```python
from build123d import *

# Parameters (mm, degrees)
SKETCH_1_W          = 56
SKETCH_1_H          = 56
EXTRUDE_1_DEPTH     = 55
SKETCH_2_W          = 9
SKETCH_2_H          = 9
CUT_EXTRUDE_1_DEPTH = 49
FILLET_1_R          = 2
SKETCH_3_R          = 19.1
EXTRUDE_2_DEPTH     = 1.6
SKETCH_4_R          = 3.175
EXTRUDE_3_DEPTH     = 18
SKETCH_5_R          = 2.5
CUT_EXTRUDE_2_DEPTH = 18
CHAMFER_1_SIZE      = 0.5


with BuildPart() as part:
    # Эскиз1 → Вытянуть1 (new body)
    with BuildSketch(Plane.XY):
        with Locations((28, 28)):
            Rectangle(SKETCH_1_W, SKETCH_1_H)
    extrude(amount=EXTRUDE_1_DEPTH)

    # Эскиз2 → Вырез-Вытянуть1 (cut)
    with BuildSketch(Plane(origin=(0, 0, 0), x_dir=(-1, 0, 0), z_dir=(0, 0, -1))):
        with Locations((-51.5, 51.5)):
            Rectangle(SKETCH_2_W, SKETCH_2_H)
        with Locations((-4.5, 51.5)):
            Rectangle(SKETCH_2_W, SKETCH_2_H)
        with Locations((-4.5, 4.5)):
            Rectangle(SKETCH_2_W, SKETCH_2_H)
        with Locations((-51.5, 4.5)):
            Rectangle(SKETCH_2_W, SKETCH_2_H)
    extrude(amount=-CUT_EXTRUDE_1_DEPTH, mode=Mode.SUBTRACT)

    # Скругление1
    fillet_1_edges = [part.edges().sort_by_distance(p)[0] for p in [
        (28, 56, 0),
        (56, 47, 24.5),
        (47, 56, 24.5),
        (47, 47, 24.5),
        (51.5, 47, 0),
        (47, 51.5, 0),
        (0, 28, 0),
        (9, 56, 24.5),
        (0, 47, 24.5),
        (9, 47, 24.5),
        (9, 51.5, 0),
        (4.5, 47, 0),
        (28, 0, 0),
        (0, 9, 24.5),
        (9, 0, 24.5),
        (9, 9, 24.5),
        (4.5, 9, 0),
        (9, 4.5, 0),
        (56, 28, 0),
        (47, 0, 24.5),
        (56, 9, 24.5),
        (47, 9, 24.5),
        (47, 4.5, 0),
        (51.5, 9, 0),
        (0, 56, 52),
        (56, 56, 52),
        (56, 0, 52),
        (0, 0, 52),
    ]]
    fillet(fillet_1_edges, radius=FILLET_1_R)

    # Эскиз3 → Вытянуть2 (add)
    with BuildSketch(Plane.XY.offset(55)):
        with Locations(Location((28, 28, 0), (0, 0, 180))):
            Circle(SKETCH_3_R)
    extrude(amount=EXTRUDE_2_DEPTH)

    # Эскиз4 → Вытянуть3 (add)
    with BuildSketch(Plane.XY.offset(56.6)):
        with Locations((28, 28)):
            Circle(SKETCH_4_R)
    extrude(amount=EXTRUDE_3_DEPTH)

    # Эскиз5 → Вырез-Вытянуть2 (cut)
    with BuildSketch(Plane.XY.offset(55)):
        with Locations((4.5, 51.5)):
            Circle(SKETCH_5_R)
        with Locations((51.5, 51.5)):
            Circle(SKETCH_5_R)
        with Locations((4.5, 4.5)):
            Circle(SKETCH_5_R)
        with Locations((51.5, 4.5)):
            Circle(SKETCH_5_R)
    extrude(amount=-CUT_EXTRUDE_2_DEPTH, mode=Mode.SUBTRACT)

    # Фаска1
    chamfer_1_edges = [part.edges().sort_by_distance(p)[0] for p in [
        (24.825, 28, 74.6),
    ]]
    chamfer(chamfer_1_edges, length=CHAMFER_1_SIZE)


solid = part.part
```
Verification items for the finished model (mm, model axes). A direction names the side the tool comes from. Coordinates: 2 decimals unless noted, no trailing zeros. Loops run counter-clockwise (first coordinate to the right, second up) from the corner with the lowest first, then second, coordinate; pieces in that order, holes last. Notation, with made-up numbers: (71.25, 86.25) -> (110.25, 86.25) arc R35 cw to (110.25, 125.25) -> close; hole circle Ø7 at (1, 54.5). An arc over 180 degrees is marked (long way). Answer in a Markdown table with one row per item. Add a question column.
1. Access from +Z, -Z, +X, -X, +Y, -Y to the whole of each face (thin tool, end or side, straight path). Record for faces 1 (the face through (46.4, 51.54, 0.57)), 2 (the face through (9, 4, 25)), 3 (the face through (46.4, 4.54, 0.57)).
2. Material ranges on probe 1 along Y at (x, z) = (51.5, 52.75); probe 2 along Y at (x, z) = (4, 51), recorded low to high. Write a range as [from, to].
3. Depth check by flat-ended pin: P1, Ø10, axis at x = 18, y = 50, coming from the +Z side; P2, Ø5.5, axis at x = 3.5, z = 21.5, coming from the +Y side; P3, Ø5.5, axis at x = 50, y = 53, coming from the -Z side. Enter the tip coordinate at first touch or a pass-through.
4. Section check A-A, the plane x = 51.5. Enter the section's corners in (y, z).
5. Section check D-D, the plane y = 28. Enter the section's corners in (x, z) (3 decimals).
6. Section check C-C, the plane z = 43. Enter the section's corners in (x, y).
7. Draft check along Y on faces 4 (the face through (55.4, 0.57, 52.04)), 5 (the face through (54.2, 4.4, 49)), 6 (the face through (53.81, 3.54, 52.04)). Enter one of: +Y half, -Y half, draft (parallel to the pull), parting line (faces both ways), or undercut.
Derived:
| question | item | result |
|---|---|---|
| 1 | face 1 | -Z, +X, +Y |
| 1 | face 2 | -Z, -X, -Y |
| 1 | face 3 | -Z, +X, -Y |
| 2 | probe 1 | y = [0, 2], [7, 49], [54, 56] |
| 2 | probe 2 | y = [0, 2.05], [6.95, 49.05], [53.95, 56] |
| 3 | P1 | stops at z = 55 |
| 3 | P2 | stops at y = 47 |
| 3 | P3 | stops at z = 49 |
| 4 | outline | (0, 49) -> (2, 49) -> (2, 55) -> (0, 55) -> close; (7, 49) -> (9, 49) -> (9, 2) arc R2 ccw to (11, 0) -> (45, 0) arc R2 ccw to (47, 2) -> (47, 49) -> (49, 49) -> (49, 55) -> (7, 55) -> close; (54, 49) -> (56, 49) -> (56, 55) -> (54, 55) -> close |
| 5 | outline | (0, 2) arc R2 ccw to (2, 0) -> (54, 0) arc R2 ccw to (56, 2) -> (56, 55) -> (47.1, 55) -> (47.1, 56.6) -> (31.175, 56.6) -> (31.175, 74.1) -> (30.675, 74.6) -> (25.325, 74.6) -> (24.825, 74.1) -> (24.825, 56.6) -> (8.9, 56.6) -> (8.9, 55) -> (0, 55) -> close |
| 6 | outline | (0, 11) arc R2 ccw to (2, 9) -> (7, 9) arc R2 cw to (9, 7) -> (9, 2) arc R2 ccw to (11, 0) -> (45, 0) arc R2 ccw to (47, 2) -> (47, 7) arc R2 cw to (49, 9) -> (54, 9) arc R2 ccw to (56, 11) -> (56, 45) arc R2 ccw to (54, 47) -> (49, 47) arc R2 cw to (47, 49) -> (47, 54) arc R2 ccw to (45, 56) -> (11, 56) arc R2 ccw to (9, 54) -> (9, 49) arc R2 cw to (7, 47) -> (2, 47) arc R2 ccw to (0, 45) -> close |
| 7 | face 4 | -Y half |
| 7 | face 5 | draft |
| 7 | face 6 | undercut |
